Could you check a few things on this model? Use its own coordinates, in mm. A direction names the side the tool comes from. Round coordinates to 2 decimals unless told otherwise and drop trailing zeros. Loops run counter-clockwise (first coordinate to the right, second up) from the corner with the lowest first, then second, coordinate; pieces in that order, holes last. Notation, with made-up numbers: (-6, -20) -> (47, -20) arc R21 cw to (47, 17) -> close; hole circle Ø4 at (38.25, 89.25). An arc over 180 degrees is marked (long way). Write each question's results on one line, items separated by ' | '. Start each with the question number.
1) Imagine slicing it at B-B, the plane y = 238.66. List the corners of the cut face in (x, z) for me.
2) Imagine slicing it at C-C, the plane z = 149. List the corners of the cut face in (x, y) for me.
3) For P1, Ø14.5, axis at x = 35, z = 147.02, coming from the -Y side; P2, Ø13, axis at x = 22.14, y = 238.66, coming from the -Z side; P3, Ø1.5, axis at x = -5, z = 128, coming from the +Y side; P4, Ø13.5, axis at y = 191.5, z = 81, coming from the +X side, each with a flat end and sliding along its axis, tell me the tip position at first contact or that it passes through.
4) Which directions (+Z, -Z, +X, -X, +Y, -Y) give clear straight access to the entire face, cutting with the end or side of a thin tool? Please do faces 4 (the flat face through (-26, 20, 146)), 5 (the flat face through (-51, 285, 112.487)), 6 (the flat face through (-85, 146, 59)), 7 (the flat face through (-31, 297, 120.487)).
5) If I drill on probe 1 along X at (y, z) = (332.94, 109.5); probe 2 along Y at (x, z) = (-72, 106); probe 3 along X at (y, z) = (332, 105), over which ranges is the centre line in solid material (lowest first)?
6) Imagine slicing it at D-D, the plane z = 53.5. List the corners of the cut face in (x, y) for me.
7) We'd pull the mould along Z, two halves only. Please class faces 1 (the cylindrical face through (24.828, 337.156, 107.557)), 2 (the flat face through (-25.1, 188.28, 90.31)), 3 (the cylindrical face through (35.53, 24.93, 135.03)): pulls with the +Z half, pulls with the -Z half, needs draft (parallel to the pull), parting line crosses it, or undercut.
8) Imagine slicing it at A-A, the plane x = -25. List the corners of the cut face in (y, z) for me.
from build123d import *
from OCP.BRepFilletAPI import BRepFilletAPI_MakeChamfer
from build123d.topology import SkipClean

# Parameters (mm, degrees)
SKETCH_1_W               = 150
SKETCH_1_H               = 150
EXTRUDE_1_DEPTH          = 20
SKETCH_2_W               = 200
SKETCH_2_H               = 170
EXTRUDE_2_DEPTH          = 20
SKETCH_3_W               = 200
SKETCH_3_H               = 22.5
EXTRUDE_3_DEPTH          = 20
SKETCH_4_W               = 200
SKETCH_4_H               = 101.536616744
SKETCH_4_R               = 12
EXTRUDE_4_DEPTH          = 10
SKETCH_5_W               = 200
SKETCH_5_H               = 170
EXTRUDE_5_DEPTH          = 10
SKETCH_6_W               = 12.361111111
SKETCH_6_H               = 120
EXTRUDE_6_DEPTH          = 60
CHAMFER_1_SIZE           = 10
CHAMFER_1_SIZE2          = 12.546778674
SKETCH_8_R               = 12.5
CUT_EXTRUDE_1_DEPTH      = 200
SKETCH_9_R               = 5.6
CUT_EXTRUDE_2_DEPTH      = 200
FILLET_1_R               = 10
SKETCH_10_R              = 40
SKETCH_10_R_2            = 8.532995409
EXTRUDE_7_DEPTH          = 5
SKETCH_11_R              = 12.5
CUT_EXTRUDE_3_DEPTH      = 200
SKETCH_12_W              = 50
SKETCH_12_H              = 12.140710291
EXTRUDE_8_DEPTH          = 120
EXTRUDE_9_DEPTH          = 120
SKETCH_14_R              = 5
SKETCH_14_R_2            = 5.6
CUT_EXTRUDE_4_DEPTH      = 200
CUT_EXTRUDE_5_DEPTH      = 428.663313117
CUT_EXTRUDE_5_DEPTH_BACK = 428.663313117
SKETCH_16_W              = 64.88929467
SKETCH_16_H              = 154.650571828
SKETCH_17_R              = 25
SKETCH_17_R_2            = 12.5
EXTRUDE_11_DEPTH         = 8
FILLET_2_R               = 10
RIB_1_REACH              = 411.018
SKETCH_18_WALL_W         = 895.028437604
SKETCH_18_WALL_H         = 15
CUT_EXTRUDE_6_DEPTH      = 425.676064177
CUT_EXTRUDE_6_DEPTH_BACK = 425.676064177
SKETCH_19_R              = 12.5


with BuildPart() as part:
    # 草图1 → 凸台-拉伸1 (new body)
    with BuildSketch(Plane(origin=(0, 0, 0), x_dir=(1, 0, 0), z_dir=(0, 1, 0))):
        Rectangle(SKETCH_1_W, SKETCH_1_H)
    extrude(amount=EXTRUDE_1_DEPTH)

    # 草图2 → 凸台-拉伸2 (add)
    with BuildSketch(Plane(origin=(0, 20, 0), x_dir=(1, 0, 0), z_dir=(0, 1, 0))):
        with Locations((-25, 0)):
            Rectangle(SKETCH_2_W, SKETCH_2_H)
    extrude(amount=-EXTRUDE_2_DEPTH)

    # 草图3 → 凸台-拉伸3 (add)
    with BuildSketch(Plane(origin=(0, 20, 0), x_dir=(1, 0, 0), z_dir=(0, 1, 0))):
        with Locations((-25, -96.25)):
            Rectangle(SKETCH_3_W, SKETCH_3_H)
    extrude(amount=-EXTRUDE_3_DEPTH)

    # 草图4 → 凸台-拉伸4 (add)
    with BuildSketch(Plane(origin=(0, 20, 0), x_dir=(1, 0, 0), z_dir=(0, 1, 0))):
        with Locations((-25, -135.768308372)):
            Rectangle(SKETCH_4_W, SKETCH_4_H)
        with Locations(Location((35, -147.018308372, 0), (0, 0, 270))):
            Circle(SKETCH_4_R, mode=Mode.SUBTRACT)
        with Locations(Location((-85, -147.018308372, 0), (0, 0, 270))):
            Circle(SKETCH_4_R, mode=Mode.SUBTRACT)
    extrude(amount=EXTRUDE_4_DEPTH)

    # 草图5 → 凸台-拉伸5 (add)
    with BuildSketch(Plane(origin=(0, 20, 0), x_dir=(1, 0, 0), z_dir=(0, 1, 0))):
        with Locations((-25, 0)):
            Rectangle(SKETCH_5_W, SKETCH_5_H)
    extrude(amount=EXTRUDE_5_DEPTH)

    # 草图6 → 凸台-拉伸6 (add, symmetric)
    with BuildSketch(Plane(origin=(-25, 0, 0), x_dir=(0, 0, -1), z_dir=(1, 0, 0))):
        Polygon((-67.5, 30), (-5, 30), (-42.777777778, 230), (-67.5, 230), align=None)
        with Locations((-61.319444445, 290)):
            Rectangle(SKETCH_6_W, SKETCH_6_H)
    extrude(amount=EXTRUDE_6_DEPTH, both=True)

    # 倒角1: one chamfer whose edges measure the first distance from different faces: ONE call of the kernel's chamfer builder (chamfer() names one face for all edges)
    chamfer_1_edges_1 = [part.edges().sort_by_distance(p)[0] for p in [
        (-85, 30, 36.25),
        (-25, 30, 67.5),
        (35, 30, 36.25),
    ]]
    chamfer_1_edges_2 = [part.edges().sort_by_distance(p)[0] for p in [
        (-25, 30, 5),
    ]]
    chamfer_1_side_2 = [part.faces().sort_by_distance(p)[0] for p in [
        (-121.627580479, 30, 50.768308372),
    ]]
    chamfer_1 = BRepFilletAPI_MakeChamfer(part.part.solid().wrapped)
    for e in chamfer_1_edges_1:
        chamfer_1.Add(CHAMFER_1_SIZE, e.wrapped)
    for e in chamfer_1_edges_2:
        chamfer_1.Add(CHAMFER_1_SIZE, CHAMFER_1_SIZE2, e.wrapped, chamfer_1_side_2[0].wrapped)  # the first distance lies on this face
    add(Compound.cast(chamfer_1.Shape()), mode=Mode.REPLACE)

    # 草图8 → 切除-拉伸1 (cut)
    with BuildSketch(Plane.XY.offset(67.5)):
        with Locations((-25, 285.8)):
            Circle(SKETCH_8_R)
    extrude(amount=-CUT_EXTRUDE_1_DEPTH, mode=Mode.SUBTRACT)

    # 草图9 → 切除-拉伸2 (cut)
    with BuildSketch(Plane.XY.offset(67.5)):
        with Locations((-72.14, 333.54)):
            Circle(SKETCH_9_R)
        with Locations((-72.14, 239.26)):
            Circle(SKETCH_9_R)
        with Locations((22.14, 239.26)):
            Circle(SKETCH_9_R)
        with Locations((22.14, 333.54)):
            Circle(SKETCH_9_R)
    extrude(amount=-CUT_EXTRUDE_2_DEPTH, mode=Mode.SUBTRACT)

    # 圆角1
    fillet_1_edges = [part.edges().sort_by_distance(p)[0] for p in [
        (35, 350, 61.319444444),
        (-85, 350, 61.319444444),
    ]]
    fillet(fillet_1_edges, radius=FILLET_1_R)

    # 草图10 → 凸台-拉伸7 (add)
    with BuildSketch(Plane.XY.offset(67.5)):
        with Locations((-25, 285.8)):
            Circle(SKETCH_10_R)
        with Locations((-25, 285.8)):
            Circle(SKETCH_10_R_2, mode=Mode.SUBTRACT)
    extrude(amount=EXTRUDE_7_DEPTH)

    # 草图11 → 切除-拉伸3 (cut)
    with BuildSketch(Plane.XY.offset(72.5)):
        with Locations((-25, 285.8)):
            Circle(SKETCH_11_R)
    extrude(amount=-CUT_EXTRUDE_3_DEPTH, mode=Mode.SUBTRACT)

    # 草图12 → 凸台-拉伸8 (add)
    with BuildSketch(Plane(origin=(35, 0, 0), x_dir=(0, 0, -1), z_dir=(1, 0, 0))):
        with Locations((-67.777777778, 223.929644855)):
            Rectangle(SKETCH_12_W, SKETCH_12_H)
    extrude(amount=-EXTRUDE_8_DEPTH)

    # 草图13 → 凸台-拉伸9 (add)
    with BuildSketch(Plane(origin=(35, 0, 0), x_dir=(0, 0, -1), z_dir=(1, 0, 0))):
        Polygon((-92.777777778, 230), (-102.486640647, 230), (-102.486640647, 350), (-112.486640647, 350), (-112.486640647, 230), (-112.486640647, 217.859289709), (-92.777777778, 217.859289709), align=None)
    extrude(amount=-EXTRUDE_9_DEPTH)

    # 草图14 → 切除-拉伸4 (cut)
    with BuildSketch(Plane.XY.offset(112.486640647)):
        with Locations((22.14, 332.94)):
            Circle(SKETCH_14_R)
        with Locations((22.14, 238.66)):
            Circle(SKETCH_14_R_2)
        with Locations((-72.14, 238.66)):
            Circle(SKETCH_14_R_2)
        with Locations((-72.14, 332.94)):
            Circle(SKETCH_14_R_2)
    extrude(amount=-CUT_EXTRUDE_4_DEPTH, mode=Mode.SUBTRACT)

    # 草图16 → 切除-拉伸5 (cut, two sides: drawn at the far end of the back side and taken through both)
    with BuildSketch(Plane.ZY.offset(85).offset(-CUT_EXTRUDE_5_DEPTH_BACK)):
        with Locations((49.451016332, 307.325285914)):
            Rectangle(SKETCH_16_W, SKETCH_16_H)
    extrude(amount=CUT_EXTRUDE_5_DEPTH + CUT_EXTRUDE_5_DEPTH_BACK, mode=Mode.SUBTRACT)

    # 草图17 → 凸台-拉伸11 (add)
    with BuildSketch(Plane.XY.offset(112.486640647)):
        with Locations((-24.999999135, 285.832995409)):
            Circle(SKETCH_17_R)
        with Locations((-24.999999135, 285.832995409)):
            Circle(SKETCH_17_R_2, mode=Mode.SUBTRACT)
    extrude(amount=EXTRUDE_11_DEPTH)

    # 圆角2
    fillet_2_edges = [part.edges().sort_by_distance(p)[0] for p in [
        (35, 350, 107.486640647),
        (-85, 350, 107.486640647),
    ]]
    fillet(fillet_2_edges, radius=FILLET_2_R)

    # 草图18 wall → 筋1 (add, up to next)
    with BuildSketch(Plane(origin=(-25, 187.859289709, 89.993320324), x_dir=(0, -0.800085500873, -0.599885981911), z_dir=(0, 0.599885981911, -0.800085500873)), mode=Mode.PRIVATE) as rib_1_sk1:
        Rectangle(SKETCH_18_WALL_W, SKETCH_18_WALL_H)
    rib_1_tool1 = extrude(rib_1_sk1.sketch, amount=RIB_1_REACH, mode=Mode.PRIVATE) - part.part
    add(rib_1_tool1.solids().sort_by_distance((-25, 187.859289709, 89.993320324))[0])

    # 草图19 → 切除-拉伸6 (cut, two sides: drawn at the far end of the back side and taken through both)
    with SkipClean():  # the faces are left unmerged after this step: merging them gives an invalid solid
        with BuildSketch(Plane.XY.offset(120.486640647).offset(-CUT_EXTRUDE_6_DEPTH_BACK)):
            with Locations(Location((-24.999999135, 285.832995409, 0), (0, 0, 180))):
                Circle(SKETCH_19_R)
        extrude(amount=CUT_EXTRUDE_6_DEPTH + CUT_EXTRUDE_6_DEPTH_BACK, mode=Mode.SUBTRACT)
    add(part.part.scale(1), mode=Mode.REPLACE)  # the faces are merged on a copy


solid = part.part
Checked values:
1) outline: (-85, 102.49) -> (-77.74, 102.49) -> (-77.74, 112.49) -> (-85, 112.49) -> close; (-66.54, 102.49) -> (16.54, 102.49) -> (16.54, 112.49) -> (-66.54, 112.49) -> close; (27.74, 102.49) -> (35, 102.49) -> (35, 112.49) -> (27.74, 112.49) -> close
2) outline: (-125, 20) -> (-96.84, 20) -> (-96.84, 30) -> (-125, 30) -> close; (-73.16, 20) -> (23.16, 20) -> (23.16, 30) -> (-73.16, 30) -> close; (46.84, 20) -> (75, 20) -> (75, 30) -> (46.84, 30) -> close
3) P1: through | P2: z = 102.49 | P3: y = 30 | P4: x = -17.5
4) face 4: +Z, +X, -X, -Y | face 5: +Z | face 6: +Z, -Z, -X, +Y | face 7: +Z, +X, -X, +Y
5) probe 1: -85 to -77.74, -66.54 to 17.14, 27.14 to 35 | probe 2: 0 to 30, 217.86 to 233.06, 244.26 to 327.34, 338.54 to 350 | probe 3: -85 to -77.66, -66.62 to 17.23, 27.05 to 35
6) outline: (-125, 0) -> (75, 0) -> (75, 30) -> (45, 30) -> (35, 40) -> (35, 230) -> (-85, 230) -> (-85, 40) -> (-95, 30) -> (-125, 30) -> close
7) face 1: needs draft | face 2: pulls with the +Z half | face 3: undercut
8) outline: (0, -85) -> (30, -85) -> (30, -5) -> (42.33, 7.33) -> (230, 42.78) -> (230, 102.49) -> (273.33, 102.49) -> (273.33, 120.49) -> (260.83, 120.49) -> (260.83, 112.49) -> (217.86, 112.49) -> (157.86, 67.5) -> (40, 67.5) -> (30, 77.5) -> (30, 186.54) -> (20, 186.54) -> (20, 107.5) -> (0, 107.5) -> close; (298.33, 102.49) -> (350, 102.49) -> (350, 112.49) -> (310.83, 112.49) -> (310.83, 120.49) -> (298.33, 120.49) -> close
